```python
from build123d import *

# Parameters (mm, degrees)
EXTRUDE_1_DEPTH     = 5
SKETCH_2_R          = 1.5
CUT_EXTRUDE_1_DEPTH = 19
SKETCH_3_R          = 40.5
EXTRUDE_2_DEPTH     = 15
EXTRUDE_3_DEPTH     = 1
SKETCH_7_W          = 0.4
SKETCH_7_H          = 0.4
SKETCH_7_W_2        = 0.2
SKETCH_7_H_2        = 0.8
EXTRUDE_4_DEPTH     = 7
SKETCH_8_R          = 1.65
SKETCH_8_R_2        = 1.5
CUT_EXTRUDE_2_DEPTH = 0.5
CUT_EXTRUDE_3_DEPTH = 0.5


with BuildPart() as part:
    # 草图1 → 凸台-拉伸1 (new body)
    with BuildSketch(Plane.XY):
        with BuildLine():
            Line((-20.976176963, 41.5), (20.976176963, 41.5))
            ThreePointArc((20.976176963, 41.5), (32.880465325, 32.880465325), (41.5, 20.976176963))
            Line((41.5, 20.976176963), (41.5, -20.976176963))
            ThreePointArc((41.5, -20.976176963), (32.880465325, -32.880465325), (20.976176963, -41.5))
            Line((20.976176963, -41.5), (-20.976176963, -41.5))
            ThreePointArc((-20.976176963, -41.5), (-32.880465325, -32.880465325), (-41.5, -20.976176963))
            Line((-41.5, -20.976176963), (-41.5, 20.976176963))
            ThreePointArc((-41.5, 20.976176963), (-32.880465325, 32.880465325), (-20.976176963, 41.5))
        make_face()
    extrude(amount=EXTRUDE_1_DEPTH)

    # 草图2 → 切除-拉伸1 (cut)
    with BuildSketch(Plane.XY.offset(5)):
        with Locations((-30.4, 30.4)):
            Circle(SKETCH_2_R)
        with Locations((30.4, 30.4)):
            Circle(SKETCH_2_R)
        with Locations((30.4, -30.4)):
            Circle(SKETCH_2_R)
        with Locations((-30.4, -30.4)):
            Circle(SKETCH_2_R)
    extrude(amount=-CUT_EXTRUDE_1_DEPTH, mode=Mode.SUBTRACT)

    # 草图3 → 凸台-拉伸2 (add)
    with BuildSketch(Plane(origin=(0, 0, 0), x_dir=(-1, 0, 0), z_dir=(0, 0, -1))):
        with Locations(Location((0, 0, 0), (0, 0, 180))):
            Circle(SKETCH_3_R)
    extrude(amount=EXTRUDE_2_DEPTH)

    # 草图6 → 凸台-拉伸3 (add)
    with BuildSketch(Plane(origin=(0, 0, -15), x_dir=(-1, 0, 0), z_dir=(0, 0, -1))):
        with BuildLine():
            Line((-18, -5.75), (-18, -7.75))
            Line((-18, -7.75), (-22, -7.75))
            Line((-22, -7.75), (-22, -5.75))
            ThreePointArc((-22, -5.75), (-21.853553391, -5.396446609), (-21.5, -5.25))
            Line((-21.5, -5.25), (-18.5, -5.25))
            ThreePointArc((-18.5, -5.25), (-18.146446609, -5.396446609), (-18, -5.75))
        make_face()
        with BuildLine():
            Line((-21.5, -8.25), (-18.5, -8.25))
            ThreePointArc((-18.5, -8.25), (-18.146446609, -8.396446609), (-18, -8.75))
            Line((-18, -8.75), (-18, -10.75))
            Line((-18, -10.75), (-22, -10.75))
            Line((-22, -10.75), (-22, -8.75))
            ThreePointArc((-22, -8.75), (-21.853553391, -8.396446609), (-21.5, -8.25))
        make_face()
        with BuildLine():
            Line((-18, -2.75), (-18, -4.75))
            Line((-18, -4.75), (-22, -4.75))
            Line((-22, -4.75), (-22, -2.75))
            ThreePointArc((-22, -2.75), (-21.853553391, -2.396446609), (-21.5, -2.25))
            Line((-21.5, -2.25), (-18.5, -2.25))
            ThreePointArc((-18.5, -2.25), (-18.146446609, -2.396446609), (-18, -2.75))
        make_face()
        with BuildLine():
            Line((-21.5, -11.25), (-18.5, -11.25))
            ThreePointArc((-18.5, -11.25), (-18.146446609, -11.396446609), (-18, -11.75))
            Line((-18, -11.75), (-18, -13.75))
            Line((-18, -13.75), (-22, -13.75))
            Line((-22, -13.75), (-22, -11.75))
            ThreePointArc((-22, -11.75), (-21.853553391, -11.396446609), (-21.5, -11.25))
        make_face()
        with BuildLine():
            Line((-22, -14.75), (-22, -16.75))
            Line((-22, -16.75), (-18, -16.75))
            Line((-18, -16.75), (-18, -14.75))
            ThreePointArc((-18, -14.75), (-18.146446609, -14.396446609), (-18.5, -14.25))
            Line((-18.5, -14.25), (-21.5, -14.25))
            ThreePointArc((-21.5, -14.25), (-21.853553391, -14.396446609), (-22, -14.75))
        make_face()
    extrude(amount=EXTRUDE_3_DEPTH)

    # 草图7 → 凸台-拉伸4 (add)
    with BuildSketch(Plane(origin=(0, 0, -16), x_dir=(-1, 0, 0), z_dir=(0, 0, -1))):
        with Locations((-19.248388447, -6.540012069)):
            Rectangle(SKETCH_7_W, SKETCH_7_H)
        with Locations((-20.931423751, -3.588755831)):
            Rectangle(SKETCH_7_W_2, SKETCH_7_H_2)
        with Locations((-19.248388447, -3.588755831)):
            Rectangle(SKETCH_7_W, SKETCH_7_H)
        with Locations((-20.931423751, -6.540012069)):
            Rectangle(SKETCH_7_W_2, SKETCH_7_H_2)
        with Locations((-19.248388447, -9.597001128)):
            Rectangle(SKETCH_7_W, SKETCH_7_H)
        with Locations((-20.931423751, -9.597001128)):
            Rectangle(SKETCH_7_W_2, SKETCH_7_H_2)
        with Locations((-20.931423751, -12.516173633)):
            Rectangle(SKETCH_7_W_2, SKETCH_7_H_2)
        with Locations((-19.248388447, -12.516173633)):
            Rectangle(SKETCH_7_W, SKETCH_7_H)
        with Locations((-19.248388447, -15.44492275)):
            Rectangle(SKETCH_7_W, SKETCH_7_H)
        with Locations((-20.931423751, -15.44492275)):
            Rectangle(SKETCH_7_W_2, SKETCH_7_H_2)
    extrude(amount=EXTRUDE_4_DEPTH)

    # 草图8 → 切除-拉伸2 (cut)
    # profile 1 of 2: a face of its own
    with BuildSketch(Plane(origin=(0, 0, -15), x_dir=(-1, 0, 0), z_dir=(0, 0, -1))):
        with Locations((-20, 0)):
            Circle(SKETCH_8_R)
        with Locations((-20, 0)):
            Circle(SKETCH_8_R_2, mode=Mode.SUBTRACT)
    # profile 2 of 2: a face of its own
    with BuildSketch(Plane(origin=(0, 0, -15), x_dir=(-1, 0, 0), z_dir=(0, 0, -1))):
        with Locations((-20, -19)):
            Circle(SKETCH_8_R)
        with Locations((-20, -19)):
            Circle(SKETCH_8_R_2, mode=Mode.SUBTRACT)
    extrude(amount=-CUT_EXTRUDE_2_DEPTH, mode=Mode.SUBTRACT)

    # 草图9 → 切除-拉伸3 (cut)
    with BuildSketch(Plane(origin=(0, 0, -15), x_dir=(-1, 0, 0), z_dir=(0, 0, -1))):
        with BuildLine():
            Line((-21.300685051, 0.747140146), (-19.096187693, -1.197131285))
            ThreePointArc((-19.096187693, -1.197131285), (-18.875022153, -0.99218186), (-18.699314949, -0.747140146))
            Line((-18.699314949, -0.747140146), (-20.903812307, 1.197131285))
            ThreePointArc((-20.903812307, 1.197131285), (-21.124977847, 0.99218186), (-21.300685051, 0.747140146))
        make_face()
        with BuildLine():
            Line((-21.300685051, -18.252859854), (-19.096187693, -20.197131285))
            ThreePointArc((-19.096187693, -20.197131285), (-18.875022153, -19.99218186), (-18.699314949, -19.747140146))
            Line((-18.699314949, -19.747140146), (-20.903812307, -17.802868715))
            ThreePointArc((-20.903812307, -17.802868715), (-21.124977847, -18.00781814), (-21.300685051, -18.252859854))
        make_face()
    extrude(amount=-CUT_EXTRUDE_3_DEPTH, mode=Mode.SUBTRACT)


solid = part.part
```
Work out the finished part from the listing and answer in its coordinate system (mm). A direction names the side the tool comes from. Coordinates: 2 decimals unless noted, no trailing zeros. Loops run counter-clockwise (first coordinate to the right, second up) from the corner with the lowest first, then second, coordinate; pieces in that order, holes last. Notation, with made-up numbers: M 89.5,-39 L 131.5,-39 A27 cw 131.5,-10 Z; hole C 15.5,12.25 d2. An arc over 180 degrees is marked long. Use CSV: the item, a comma, the result in double quotes. Start each with the question number.
(1) Given pin 1 Ø0.6 at (y, z) = (-9.5, -19) entering from +X; pin 2 Ø6 at (y, z) = (14, -15) entering from +X; pin 3 Ø3 at (x, z) = (32, -13) entering from -Y; pin 4 Ø12 at (y, z) = (-1, -1.5) entering from +X, each flat-ended and moving along its own axis, determine where each tip first touches the part or whether it passes through.
(2) Consider line 1 (Y direction, x = 30.4, z = 1.55); line 2 (X direction, y = -3.5, z = -16.25); line 3 (Z direction, x = -11.5, y = 37). Determine where each line is inside the solid, lowest interval first.
(3) For faces 5 (the face through (38.63, -12.17, -7.4)), 6 (the face through (-31.6, 29.5, 2.5)), 7 (the face through (20.5, -0.6, -15)), determine the directions among +Z, -Z, +X, -X, +Y, -Y from which every point of the face is accessible in a straight line to the end or side of a thin tool.
(4) Find section A-A, the plane y = -30.4. Give the vertices of the cut face in (x, z), then the cut area to 3 significant figures.
(5) For a pull along X with two mould halves and no side action, classify faces 1 (the face through (19.4, -18.4, -15)), 2 (the face through (20, 0, -14.5)), 3 (the face through (19.786, -18.789, -14.754)), 4 (the face through (-33.03, 32.73, 2.46)) as +X half, -X half, draft (parallel to the pull), parting line (faces both ways), or undercut.
(6) Find section D-D, the plane y = 10. Give the vertices of the cut face in (x, z).
(7) Find section B-B, the plane x = 0. Give the vertices of the cut face in (y, z), then the cut area to 3 significant figures.
(8) Find section C-C, the plane z = -20. State how many separate pieces and enclosed holes the cut face has, then the cut area to 3 significant figures.
Recorded:
1,pin 1,"stops at x = 21.03"
1,pin 2,"stops at x = 38.98"
1,pin 3,"stops at y = -26.65"
1,pin 4,"stops at x = 41.5"
2,line 1,"y = -35.19 to -31.9, -28.9 to 28.9, 31.9 to 35.19"
2,line 2,"x = 19.05 to 19.45, 20.83 to 21.03"
2,line 3,"z = -15 to 5"
3,face 5,"-Z"
3,face 6,"+Z, -Z"
3,face 7,"-Z, +X, -X, +Y"
4,outline,"M -35.19,0 L -31.9,0 L -31.9,5 L -35.19,5 Z; M -28.9,0 L -26.76,0 L -26.76,-15 L 26.76,-15 L 26.76,0 L 28.9,0 L 28.9,5 L -28.9,5 Z; M 31.9,0 L 35.19,0 L 35.19,5 L 31.9,5 Z"
4,area,"1,120 mm^2"
5,face 1,"draft"
5,face 2,"undercut"
5,face 3,"undercut"
5,face 4,"-X half"
6,outline,"M -41.5,0 L -39.25,0 L -39.25,-15 L 39.25,-15 L 39.25,0 L 41.5,0 L 41.5,5 L -41.5,5 Z"
7,outline,"M -41.5,0 L -40.5,0 L -40.5,-15 L 40.5,-15 L 40.5,0 L 41.5,0 L 41.5,5 L -41.5,5 Z"
7,area,"1,630 mm^2"
8,separate pieces,"10"
8,enclosed holes,"0"
8,area,"1.60 mm^2"
